```python
from build123d import *

# Parameters (mm, degrees)
SKETCH1_R           = 2.1
BOSS_EXTRUDE1_DEPTH = 15
SKETCH2_W           = 82
SKETCH2_H           = 82
CUT_EXTRUDE1_DEPTH  = 10
CUT_EXTRUDE2_DEPTH  = 257.934619876


with BuildPart() as part:
    # Sketch1 → Boss-Extrude1 (new body)
    with BuildSketch(Plane(origin=(0, 0, 0), x_dir=(1, 0, 0), z_dir=(0, 1, 0))):
        with BuildLine():
            Line((-40, 117), (40, 117))
            add(Edge.make_bspline(
                [(105, 85), (82.19875176, 117.821973651), (40, 117)],
                knots=[0, 0, 0, 1, 1, 1], degree=2))
            ThreePointArc((105, 85), (99.142135624, 70.857864376), (85, 65))
            Line((85, 65), (40, 65))
            Line((40, 65), (40, -65))
            Line((40, -65), (85, -65))
            ThreePointArc((85, -65), (99.142135624, -70.857864376), (105, -85))
            add(Edge.make_bspline(
                [(105, -85), (82.19875176, -117.821973651), (40, -117)],
                knots=[0, 0, 0, 1, 1, 1], degree=2))
            Line((40, -117), (-40, -117))
            add(Edge.make_bspline(
                [(-105, -85), (-82.19875176, -117.821973651), (-40, -117)],
                knots=[0, 0, 0, 1, 1, 1], degree=2))
            ThreePointArc((-105, -85), (-99.142135624, -70.857864376), (-85, -65))
            Line((-85, -65), (-40, -65))
            Line((-40, -65), (-40, 65))
            Line((-40, 65), (-85, 65))
            ThreePointArc((-85, 65), (-99.142135624, 70.857864376), (-105, 85))
            add(Edge.make_bspline(
                [(-105, 85), (-82.19875176, 117.821973651), (-40, 117)],
                knots=[0, 0, 0, 1, 1, 1], degree=2))
        make_face()
        with Locations(Location((-85, 85, 0), (0, 0, 270))):
            Circle(SKETCH1_R, mode=Mode.SUBTRACT)
        with Locations(Location((85, 85, 0), (0, 0, 90))):
            Circle(SKETCH1_R, mode=Mode.SUBTRACT)
        with Locations(Location((-85, -85, 0), (0, 0, 90))):
            Circle(SKETCH1_R, mode=Mode.SUBTRACT)
        with Locations(Location((85, -85, 0), (0, 0, 270))):
            Circle(SKETCH1_R, mode=Mode.SUBTRACT)
    extrude(amount=BOSS_EXTRUDE1_DEPTH)

    # Sketch2 → Cut-Extrude1 (cut)
    with BuildSketch(Plane.XZ):
        Rectangle(SKETCH2_W, SKETCH2_H)
    extrude(amount=-CUT_EXTRUDE1_DEPTH, mode=Mode.SUBTRACT)

    # Sketch3 → Cut-Extrude2 (cut, through all)
    with BuildSketch(Plane(origin=(0, 0, -117), x_dir=(-1, 0, 0), z_dir=(0, 0, -1))):
        with BuildLine():
            Line((-75.688086791, 8.8904517), (-105, 8.8904517))
            Line((-105, 8.8904517), (-105, 15))
            Line((-105, 15), (-40, 15))
            add(Edge.make_bspline(
                [(-75.688086791, 8.8904517), (-63.128326114, 7.187324041), (-52.082553879, 13.673406614), (-40, 15)],
                knots=[0, 0, 0, 0, 1, 1, 1, 1], degree=3))
        make_face()
        with BuildLine():
            Line((105, 15), (40, 15))
            add(Edge.make_bspline(
                [(75.688086791, 8.8904517), (63.128326114, 7.187324041), (52.082553879, 13.673406614), (40, 15)],
                knots=[0, 0, 0, 0, 1, 1, 1, 1], degree=3))
            Line((75.688086791, 8.8904517), (105, 8.8904517))
            Line((105, 8.8904517), (105, 15))
        make_face()
    extrude(amount=-CUT_EXTRUDE2_DEPTH, mode=Mode.SUBTRACT)


solid = part.part
```
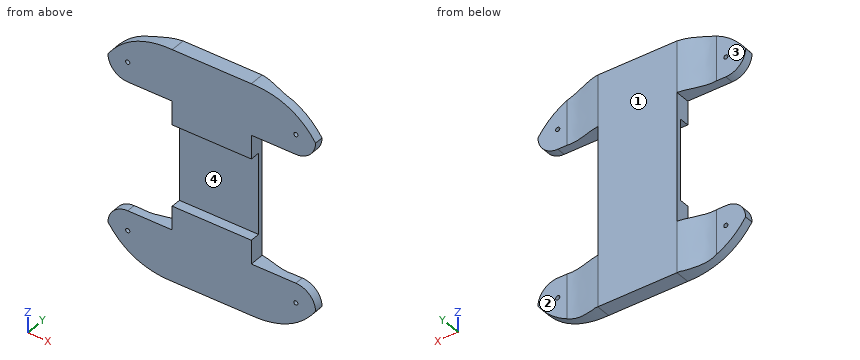
Source: CAD feature listing. Evaluate the final solid. Frame: model axes, mm. Face numbers are marked on the shaded views. A direction names the side the tool comes from. Coordinates: 2 decimals unless noted, no trailing zeros. Loops run counter-clockwise (first coordinate to the right, second up) from the corner with the lowest first, then second, coordinate; pieces in that order, holes last. Notation, with made-up numbers: M -32,20 L 14,20 A31 cw 14,57 Z; hole C 47,70 d3. An arc over 180 degrees is marked long. Put each result on its own line as item: value. Start each with the question number.
1) Ray query, L1, parallel to X at y = 6, z = -85; L2, parallel to Z at x = -85, y = 6.75; L3, parallel to Z at x = 43, y = 11.75. Return the intervals inside material, ascending. Write a range as from..to.
2) Contact query for flat-ended pins moving along their axis: pin 1 Ø6.5 at (x, z) = (-85, 85) entering from -Y; pin 2 Ø4.5 at (y, z) = (9, -1) entering from -X; pin 3 Ø1 at (x, y) = (-21, 8.5) entering from -Z; pin 4 Ø6 at (x, y) = (45.5, 3.5) entering from +Z. Output: stop coordinate, or through.
3) Reachability of the marked faces 1, 2, 3 and 4 from +Z, -Z, +X, -X, +Y, -Y: full face, straight path, thin tool, end or side. Return the list, or none.
4) Cut plane A-A on z = -11.5. Return the cut outline in (x, y).
The answers:
1. L1: x = -105..-87.1, -82.9..82.9, 87.1..105
1. L2: z = -105..-87.1, -82.9..-65, 65..82.9, 87.1..105
1. L3: z = -117.02..-65, 65..117.02
2. pin 1: stops at y = 0
2. pin 2: stops at x = -40
2. pin 3: stops at z = -117
2. pin 4: stops at z = 117.02
3. face 1: +Z, -Z, +X, -X, +Y
3. face 2: +Z, -Z, +X, +Y
3. face 3: +Z, -Z, -X, +Y
3. face 4: +X, -X, -Y
4. outline: M -40,10 L 40,10 L 40,15 L -40,15 Z
